```python
from build123d import *

# Parameters (mm, degrees)
SKETCH1_W           = 65
SKETCH1_H           = 10
BOSS_EXTRUDE1_DEPTH = 25
SKETCH2_R           = 3.5
CUT_EXTRUDE1_DEPTH  = 25
FILLET1_R           = 5


with BuildPart() as part:
    # Sketch1 → Boss-Extrude1 (new body)
    with BuildSketch(Plane(origin=(0, 0, 0), x_dir=(1, 0, 0), z_dir=(0, 1, 0))):
        with Locations((2.312734082, 5.346441948)):
            Rectangle(SKETCH1_W, SKETCH1_H)
    extrude(amount=BOSS_EXTRUDE1_DEPTH)

    # Sketch2 → Cut-Extrude1 (cut)
    with BuildSketch(Plane(origin=(0, 0, -10.346441948), x_dir=(-1, 0, 0), z_dir=(0, 0, -1))):
        with Locations((18.187265918, 19)):
            Circle(SKETCH2_R)
        with BuildLine():
            Line((-3.812734082, 17.077006126), (-3.812734082, 5.696172333))
            ThreePointArc((-3.812734082, 5.696172333), (-2.312734082, 4.196172333), (-0.812734082, 5.696172333))
            Line((-0.812734082, 5.696172333), (-0.812734082, 17.077006126))
            ThreePointArc((-0.812734082, 17.077006126), (-2.312734082, 18.577006126), (-3.812734082, 17.077006126))
        make_face()
        with Locations((-22.812734082, 19)):
            Circle(SKETCH2_R)
    extrude(amount=-CUT_EXTRUDE1_DEPTH, mode=Mode.SUBTRACT)

    # Fillet1
    fillet1_edges = [part.edges().sort_by_distance(p)[0] for p in [
        (34.812734082, 25, -5.346441948),
        (-30.187265918, 25, -5.346441948),
        (34.812734082, 0, -5.346441948),
        (-30.187265918, 0, -5.346441948),
    ]]
    fillet(fillet1_edges, radius=FILLET1_R)


solid = part.part
```
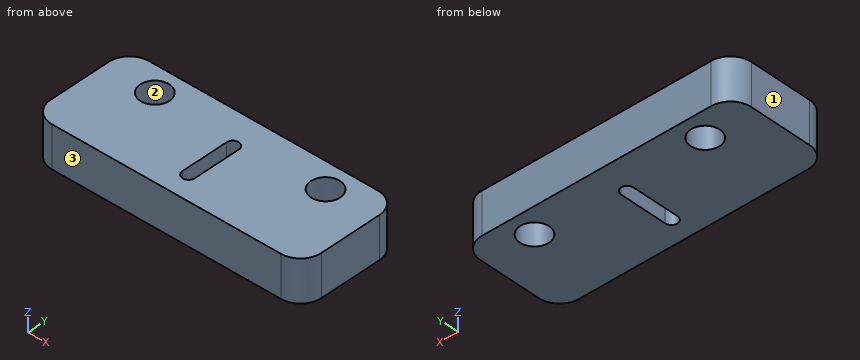
Geometry: final body of the model. Coordinates: model frame, mm. Face numbers are marked on the shaded views. Coordinates: 2 decimals unless noted, no trailing zeros. Order: outer loops, then holes, each group sorted by start corner. A loop starts at its lowest first (then second) coordinate and runs counter-clockwise, first axis right, second up. Notation, with made-up numbers: M -19.5,56 L 1.5,56 A11 cw 1.5,64 Z; hole C -11,85 d11. An arc over 180 degrees is marked long. Answer in a Markdown table with one row per item. Add a question column.
Q1. Section query A-A on y = 9.25. Return the cut outline in (x, z), and give its area (3 significant figures).
Q2. Contact query for a flat-ended pin moving along its axis: P1, Ø5.5, axis at x = 22.81, y = 19, coming from the -Z side. Output: stop coordinate, or through.
Q3. Section query B-B on z = -8.25. Return the cut outline in (x, y), and give its area (3 significant figures).
Q4. Section query C-C on x = 3. Return the cut outline in (y, z), and give its area (3 significant figures).
Q5. Line query: L1, parallel to X at y = 7.5, z = -3.75; L2, parallel to Y at x = 23, z = -6.75; L3, parallel to X at y = 5, z = -7.75. Output: solid intervals per line, ascending.
Q6. Mould query, pull axis Y, two halves, no side actions, for the marked faces 1, 2 and 3. Classes: released by +Y, released by -Y, zero draft, split by the parting line, or undercut.
Completed:
| question | item | result |
|---|---|---|
| 1 | outline | M -30.19,-10.35 L 0.81,-10.35 L 0.81,-0.35 L -30.19,-0.35 Z; M 3.81,-10.35 L 34.81,-10.35 L 34.81,-0.35 L 3.81,-0.35 Z |
| 1 | area | 620 mm2 |
| 2 | P1 | passes through |
| 3 | outline | M -30.19,5 A5 ccw -25.19,0 L 29.81,0 A5 ccw 34.81,5 L 34.81,20 A5 ccw 29.81,25 L -25.19,25 A5 ccw -30.19,20 Z; hole C -18.19,19 d7; hole M 0.81,5.7 A1.5 ccw 3.81,5.7 L 3.81,17.08 A1.5 ccw 0.81,17.08 Z; hole C 22.81,19 d7 |
| 3 | area | 1,490 mm2 |
| 4 | outline | M 0,-10.35 L 4.36,-10.35 L 4.36,-0.35 L 0,-0.35 Z; M 18.41,-10.35 L 25,-10.35 L 25,-0.35 L 18.41,-0.35 Z |
| 4 | area | 110 mm2 |
| 5 | L1 | x = -30.19 to 0.81, 3.81 to 34.81 |
| 5 | L2 | y = 0 to 15.51, 22.49 to 25 |
| 5 | L3 | x = -30.19 to 0.98, 3.64 to 34.81 |
| 6 | face 1 | zero draft |
| 6 | face 2 | undercut |
| 6 | face 3 | released by -Y |
